from build123d import *

# Parameters (mm, degrees)
EXTRUDE_START         = -360
EXTRUDE_1_DEPTH       = 12
EXTRUDE_START_2       = 28
EXTRUDE_2_DEPTH       = 10
EXTRUDE_START_3       = -38
EXTRUDE_3_DEPTH       = 10
EXTRUDE_START_4       = -46
EXTRUDE_SKETCH_4_W    = 10
EXTRUDE_SKETCH_4_H    = 56
EXTRUDE_4_DEPTH       = 92
REVOLVE_PROFILE_1_W   = 29.65
REVOLVE_PROFILE_1_H   = 80
REVOLVE_1_ANGLE       = 179
REVOLVE_INDEX_1_ANGLE = 90.5
EXTRUDE_START_5       = -32
EXTRUDE_SKETCH_5_W    = 13.5
EXTRUDE_SKETCH_5_H    = 20
EXTRUDE_5_DEPTH       = 64
EXTRUDE_SKETCH_6_W    = 13.5
EXTRUDE_SKETCH_6_H    = 20
EXTRUDE_6_DEPTH       = 64


with BuildPart() as part:
    # Extrude sketch 1 → Extrude 1 (new body)
    with BuildSketch(Plane(origin=(0, 0, 0), x_dir=(0, 0, -1), z_dir=(1, 0, 0)).offset(EXTRUDE_START)):
        with BuildLine():
            Line((-90, 96), (-90, -96))
            ThreePointArc((-90, -96), (-85.899494937, -105.899494937), (-76, -110))
            Line((-76, -110), (76, -110))
            ThreePointArc((76, -110), (85.899494937, -105.899494937), (90, -96))
            Line((90, -96), (90, 96))
            ThreePointArc((90, 96), (85.899494937, 105.899494937), (76, 110))
            Line((76, 110), (-76, 110))
            ThreePointArc((-76, 110), (-85.899494937, 105.899494937), (-90, 96))
        make_face()
    extrude(amount=EXTRUDE_1_DEPTH)


with BuildPart() as body_2:
    # Extrude sketch 2 → Extrude 2 (new body)
    with BuildSketch(Plane(origin=(0, 0, 0), x_dir=(1, 0, 0), z_dir=(0, 1, 0)).offset(EXTRUDE_START_2)):
        Polygon((-349, 80), (-48, 36), (-48, -36), (-349, -80), align=None)
    extrude(amount=EXTRUDE_2_DEPTH)


with BuildPart() as body_3:
    # Extrude sketch 3 → Extrude 3 (new body)
    with BuildSketch(Plane(origin=(0, 0, 0), x_dir=(1, 0, 0), z_dir=(0, 1, 0)).offset(EXTRUDE_START_3)):
        Polygon((-349, 80), (-48, 36), (-48, -36), (-349, -80), align=None)
    extrude(amount=EXTRUDE_3_DEPTH)


with BuildPart() as body_4:
    # Extrude sketch 4 → Extrude 4 (new body)
    with BuildSketch(Plane.XY.offset(EXTRUDE_START_4)):
        with Locations((-257, 0)):
            Rectangle(EXTRUDE_SKETCH_4_W, EXTRUDE_SKETCH_4_H)
    extrude(amount=EXTRUDE_4_DEPTH)


with BuildPart() as body_5:
    # Revolve profile 1 → Revolve 1 (revolve)
    with BuildSketch(Plane(origin=(0, 0, 0), x_dir=(1, 0, 0), z_dir=(0, 1, 0))):
        with Locations((45.175, 0)):
            Rectangle(REVOLVE_PROFILE_1_W, REVOLVE_PROFILE_1_H)
    revolve(axis=Axis((0, 0, -45), (0, 0, 1)), revolution_arc=REVOLVE_1_ANGLE)


with BuildPart() as body_5_1:
    # Revolve index 1: moved
    add(body_5.part.rotate(Axis((0, 0, 0), (0, 0, 1)), REVOLVE_INDEX_1_ANGLE))


with BuildPart() as body_6:
    # Extrude sketch 5 → Extrude 5 (new body)
    with BuildSketch(Plane.XY.offset(EXTRUDE_START_5)):
        with Locations((-7.25, 66)):
            Rectangle(EXTRUDE_SKETCH_5_W, EXTRUDE_SKETCH_5_H)
    extrude(amount=EXTRUDE_5_DEPTH)


with BuildPart() as body_7:
    # Extrude sketch 6 → Extrude 6 (new body)
    with BuildSketch(Plane.XY.offset(EXTRUDE_START_5)):
        with Locations((-7.25, -66)):
            Rectangle(EXTRUDE_SKETCH_6_W, EXTRUDE_SKETCH_6_H)
    extrude(amount=EXTRUDE_6_DEPTH)

    # Combine (weld / assembly of features): union body 2, body 5, body 3, body 4, body 6, part
    add(body_2.part)
    add(body_5_1.part)
    add(body_3.part)
    add(body_4.part)
    add(body_6.part)
    add(part.part)


solid = body_7.part
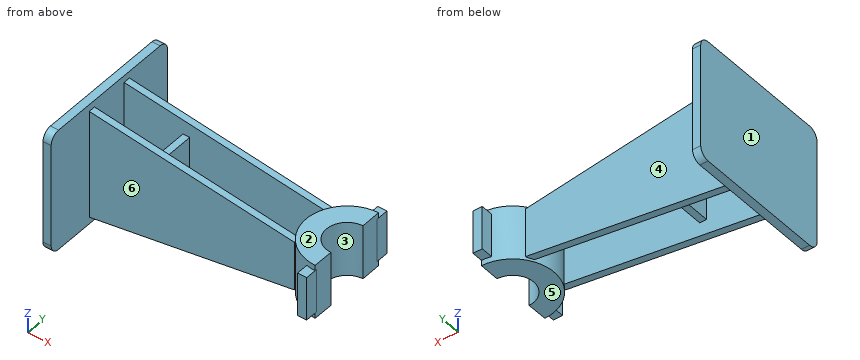
Here's how the part is built. I have some questions about the finished solid (model axes, mm). Face numbers are marked on the shaded views. A direction names the side the tool comes from. Coordinates: 2 decimals unless noted, no trailing zeros. Order: outer loops, then holes, each group sorted by start corner. A loop starts at its lowest first (then second) coordinate and runs counter-clockwise, first axis right, second up. Notation, with made-up numbers: (-16.5, 31.25) -> (7.5, 31.25) arc R10 cw to (7.5, 46.25) -> close; hole circle Ø5 at (-2, 16.25). An arc over 180 degrees is marked (long way). Answer in a Markdown table with one row per item.
(1) I want a section at B-B on z = 6.5. List the corners of the cut face in (x, y) for me, then the cut area to 3 significant figures.
Answer key:
| item | result |
|---|---|
| outline | (-360, -110) -> (-348, -110) -> (-348, -38) -> (-48, -38) -> (-48, -36) arc R60 ccw to (-14, -58.34) -> (-14, -76) -> (-0.5, -76) -> (-0.5, -57.29) -> (-0.26, -30.35) arc R30.35 cw to (-0.26, 30.35) -> (-0.5, 57.29) -> (-0.5, 76) -> (-14, 76) -> (-14, 58.34) arc R60 ccw to (-48, 36) -> (-48, 38) -> (-348, 38) -> (-348, 110) -> (-360, 110) -> close; hole (-348, -28) -> (-262, -28) -> (-262, 28) -> (-348, 28) -> close; hole (-252, -28) -> (-53.07, -28) arc R60 cw to (-53.07, 28) -> (-252, 28) -> close |
| area | 13,800 mm^2 |
(2) I want a section at C-C on x = -218.5. List the corners of the cut face in (y, z) for me.
Answer key:
| item | result |
|---|---|
| outline | (-38, -60.92) -> (-28, -60.92) -> (-28, 60.92) -> (-38, 60.92) -> close; (28, -60.92) -> (38, -60.92) -> (38, 60.92) -> (28, 60.92) -> close |
(3) I want a section at A-A on y = 0. List the corners of the cut face in (x, z) for me, then the cut area to 3 significant figures.
Answer key:
| item | result |
|---|---|
| outline | (-360, -90) -> (-348, -90) -> (-348, 90) -> (-360, 90) -> close; (-262, -46) -> (-252, -46) -> (-252, 46) -> (-262, 46) -> close; (-60, -40) -> (-30.35, -40) -> (-30.35, 40) -> (-60, 40) -> close |
| area | 5,450 mm^2 |
(4) Thinking about a two-plate mould opening in Y: for the marked faces 3, 4, 5 and 6, which applies, +Y half, -Y half, draft (parallel to the pull), parting line (faces both ways), or undercut?
Answer key:
| item | result |
|---|---|
| face 3 | undercut |
| face 4 | +Y half |
| face 5 | draft |
| face 6 | -Y half |
(5) Please list where these lines run through material, in increasing order: probe 1 along X at (y, z) = (65, -31); probe 2 along Y at (x, z) = (-89, 39.5); probe 3 along X at (y, z) = (-10, -44.5).
Answer key:
| item | result |
|---|---|
| probe 1 | -360 to -348, -14 to -0.5 |
| probe 2 | -38 to -28, 28 to 38 |
| probe 3 | -360 to -348, -262 to -252 |
(6) Will these pins go through, and if not, where does the flat tip stop? pin 1 Ø1 at (y, z) = (37, 12.5) entering from +X; pin 2 Ø8 at (y, z) = (-81.5, 23.5) entering from +X; pin 3 Ø17 at (y, z) = (-5.5, -15) entering from +X.
Answer key:
| item | result |
|---|---|
| pin 1 | x = -0.32 |
| pin 2 | x = -348 |
| pin 3 | x = -26.93 |
(7) I want a section at D-D on y = -52. List the corners of the cut face in (x, z) for me.
Answer key:
| item | result |
|---|---|
| outline | (-360, -90) -> (-348, -90) -> (-348, 90) -> (-360, 90) -> close; (-29.93, -40) -> (-0.45, -40) -> (-0.45, 40) -> (-29.93, 40) -> close |
(8) On a 3-axis mill with a long thin cutter (end or side, diameter ignored), from which of +Z, -Z, +X, -X, +Y, -Y can I reach the whole of each face in a straight line? I mean the marked faces 1 and 2. Say none if no direction works.
Answer key:
| item | result |
|---|---|
| face 1 | +Z, -Z, -X, +Y, -Y |
| face 2 | +Z, +X, +Y, -Y |
